```python
from build123d import *

# Parameters (mm, degrees)
F0_R     = 13.25
F1_DEPTH = 3.5
F2_W     = 6.9995252416
F2_H     = 11.4660244435
F3_DEPTH = 5
F4_R     = 1.115966898
F5_DEPTH = 7.5
F6_R     = 1
F7_R     = 1


with BuildPart() as f1:
    # F0 (on Top) → F1 (new body)
    with BuildSketch(Plane.XY):
        Circle(F0_R)
    extrude(amount=F1_DEPTH)

    # F2 (on face) → F3 (join)
    with BuildSketch(Plane(origin=(0, 0, 0), x_dir=(1, 0, 0), z_dir=(0, 0, -1))):
        Rectangle(F2_W, F2_H)
    extrude(amount=F3_DEPTH)

    # F4 (on Right) → F5 (join, symmetric)
    with BuildSketch(Plane.YZ):
        with Locations((0, -2.5976826437)):
            Circle(F4_R)
    extrude(amount=F5_DEPTH, both=True)

    # F6
    f6_edges = [f1.edges().sort_by_distance(p)[0] for p in [
        (-13.25, 0, 0),
    ]]
    fillet(f6_edges, radius=F6_R)

    # F7
    f7_edges = [f1.edges().sort_by_distance(p)[0] for p in [
        (0, 5.733012, -5),
        (3.499763, 0, -5),
        (0, -5.733012, -5),
        (-3.499763, 0, -5),
    ]]
    fillet(f7_edges, radius=F7_R)


solid = f1.part
```
CAD build for the part. Positions are in the model's coordinates, mm. A direction names the side the tool comes from. Coordinates: 2 decimals unless noted, no trailing zeros. Order: outer loops, then holes, each group sorted by start corner. A loop starts at its lowest first (then second) coordinate and runs counter-clockwise, first axis right, second up. Notation, with made-up numbers: M 8.5,-32 L 27.5,-32 A24 cw 27.5,-7 Z; hole C -16,82 d3. An arc over 180 degrees is marked long. Answer as CSV lines item,"result".
1) Cut at C-C (z = -0.5). List the corners of the cut face in (x, y), then the cut area to 3 significant figures.
Verdict:
outline,"M -3.5,-5.73 L 3.5,-5.73 L 3.5,5.73 L -3.5,5.73 Z"
area,"80.3 mm2"
2) Drill centre lines: L1, parallel to X at y = 0.5, z = -2.25; L2, parallel to Z at x = -4.5, y = -4.5; L3, parallel to Y at x = 0.25, z = -1.5. Where is each one in solid material? Low to high. Write a range as from..to.
Verdict:
L1,"-7.5..7.5"
L2,"0..3.5"
L3,"-5.73..5.73"
3) Mould opens along Z. For faces 1 (the cylindrical face through (-5.472, -0.242, -3.687)), 2 (the flat face through (0, -5.733, -2)), 3 (the cylindrical face through (-3.215, -0.08, -4.699)), 4 (the cylindrical face through (5.528, -0.242, -3.687)) say: released by +Z, released by -Z, zero draft, split by the parting line, or undercut.
Verdict:
face 1,"undercut"
face 2,"zero draft"
face 3,"released by -Z"
face 4,"undercut"
4) Flat gauge pins, fed straight in: P1, Ø1.5, axis at y = -9, z = 0, coming from the +X side; P2, Ø4.5, axis at y = -2.5, z = -1.5, coming from the +X side; P3, Ø1.1, axis at y = 0, z = -3, coming from the +X side. Where does each tip first touch, or does it go through?
Verdict:
P1,"x = 10.04"
P2,"x = 13.06"
P3,"x = 7.5"
5) Cut at B-B (y = 0). List the corners of the cut face in (x, z).
Verdict:
outline,"M -13.25,1 A1 ccw -12.25,0 L -3.5,0 L -3.5,-1.48 L -7.5,-1.48 L -7.5,-3.71 L -3.5,-3.71 L -3.5,-4 A1 ccw -2.5,-5 L 2.5,-5 A1 ccw 3.5,-4 L 3.5,-3.71 L 7.5,-3.71 L 7.5,-1.48 L 3.5,-1.48 L 3.5,0 L 12.25,0 A1 ccw 13.25,1 L 13.25,3.5 L -13.25,3.5 Z"
6) 3-axis set-ups, long thin cutter, end or side, ignore diameter. For faces 5 (the flat face through (0, 5.733, -2)), 6 (the flat face through (0, 0, 3.5)), 7 (the flat face through (0, 0, -5)), 8 (the flat face through (7.5, 0, -3)), 9 (the flat face through (-7.5, 0, -3)): which of +Z, -Z, +X, -X, +Y, -Y reach the whole face in a straight line?
Verdict:
face 5,"-Z, +X, -X, +Y"
face 6,"+Z, +X, -X, +Y, -Y"
face 7,"-Z, +X, -X, +Y, -Y"
face 8,"-Z, +X, +Y, -Y"
face 9,"-Z, -X, +Y, -Y"
7) Cut at A-A (x = 0). List the corners of the cut face in (y, z).
Verdict:
outline,"M -13.25,1 A1 ccw -12.25,0 L -5.73,0 L -5.73,-4 A1 ccw -4.73,-5 L 4.73,-5 A1 ccw 5.73,-4 L 5.73,0 L 12.25,0 A1 ccw 13.25,1 L 13.25,3.5 L -13.25,3.5 Z"
